Can you work these out from the model? Positions are in its coordinate system, mm. A direction names the side the tool comes from. Coordinates: 2 decimals unless noted, no trailing zeros. Order: outer loops, then holes, each group sorted by start corner. A loop starts at its lowest first (then second) coordinate and runs counter-clockwise, first axis right, second up. Notation, with made-up numbers: (19.25, 76) -> (67.25, 76) arc R27 cw to (67.25, 102) -> close; hole circle Ø9 at (73.25, 86). An arc over 180 degrees is marked (long way). Return JSON: item names as keys, results as strings. Group by question number.
1) For faces 1 (the cylindrical face through (-14.9, 7.5, 7.9)), 2 (the flat face through (-2, 8, 3.75)), 3 (the flat face through (-5, 3, 0)), which set-ups out of +Z, -Z, +X, -X, +Y, -Y let a thin tool reach every point of the face, with its end or its side?
2) If we section it at A-A, the plane z = 0: Please give me the cut outline in (x, y), then the cut area to 3 significant figures.
3) If I drill on probe 1 along Z at (x, y) = (0, 8.65) (3 decimals); probe 2 along X at (y, z) = (6.15, 0); probe 3 along Z at (x, y) = (-13.4, 6.9) (3 decimals), over which ranges is the centre line in solid material (lowest first)? Write a range as from..to.
4) If we section it at C-C, the plane y = 9: Please give me the cut outline in (x, z) (3 decimals), then the cut area to 3 significant figures.
5) If we section it at B-B, the plane x = -13.4: Please give me the cut outline in (y, z) (3 decimals), then the cut area to 3 significant figures.
6) For pin 1 (5 mm diameter, centred on x = -1, z = -0.5, fed in from -Y); pin 2 (1.5 mm diameter, centred on x = -13.5, z = -7.5, fed in from +Y); pin 3 (11.5 mm diameter, centred on x = -3, z = 1, fed in from -Y); pin 4 (2 mm diameter, centred on x = -6, z = -0.5, fed in from +Y), each with a flat end and sliding along its axis, tell me the tip position at first contact or that it passes through.
Autodesk Inventor part; units mm, degrees
ref_plane "YZ Plane" through (0, 0, 0) normal (1, 0, 0) x (0, 1, 0)
ref_plane "XZ Plane" through (0, 0, 0) normal (0, 1, 0) x (-1, 0, 0)
ref_plane "XY Plane" through (0, 0, 0) normal (0, 0, 1) x (1, 0, 0)
sketch "Sketch1" plane through (0, 0, 0) normal (0, 1, 0) x (-1, 0, 0)
  circle A0 centre (7.3, 0) radius 1.55
  circle A1 centre (0, 0) radius 1.55
  line L0 (0, 10.8163) -> (0, -10.8163)
  line L1 (6.335, 0) -> (-6.335, 0)
  line L2 (-3.05, 12.16) -> (16.95, 12.16)
  line L3 (16.95, 12.16) -> (16.95, -12.16)
  line L4 (16.95, -12.16) -> (-3.05, -12.16)
  line L5 (-3.05, -12.16) -> (-3.05, 12.16)
  dimension "d0" = 3.1
  dimension "d1" = 7.3
  dimension "d2" = 1.5
  dimension "d3" = 24.32
  dimension "d4" = 20
extrude "Extrusion1" add sketch "Sketch1" along normal blind 10
sketch "Sketch2" plane through (0, 0, 0) normal (0, -1, 0) x (1, 0, 0)
  line L0 (3.05, 5.16) -> (-11.68, 5.16)
  line L1 (-11.68, 5.16) -> (-11.68, -5.16)
  line L2 (-11.68, -5.16) -> (3.05, -5.16)
  line L3 (3.05, -5.16) -> (3.05, 5.16)
  circle A0 centre (0, 0) radius 1.55
  circle A1 centre (-7.3, 0) radius 1.55
  line L4 (0, 0) -> (-7.3, 0)
  line L5 (3.05, 12.16) -> (3.05, -12.16)
  dimension "d7" = 10.32
  dimension "d8" = 4.38
extrude "Extrusion2" cut sketch "Sketch2" against normal blind 3
sketch "Sketch3" plane through (0, 10, 0) normal (0, 1, 0) x (1, 0, 0)
  circle A0 centre (-7.3, 0) radius 1.55
  circle A1 centre (0, 0) radius 1.55
  arc A2 (3.05, -2.1817) -> (3.05, 2.1817) centre (0, 0) ccw
  arc A3 (-7.3, 3.75) -> (-7.3, -3.75) centre (-7.3, 0) ccw
  line L0 (3.05, -12.16) -> (3.05, 12.16)
  line L1 (-7.3, 3.75) -> (0, 3.75)
  line L2 (-7.3, -3.75) -> (0, -3.75)
  line L3 (3.05, -2.1817) -> (3.05, 2.1817)
  line L4 (3.05, -2.1817) -> (3.05, 2.1817)
  line L5 (0, -3.75) -> (3.05, -3.75)
  line L6 (0, 3.75) -> (3.05, 3.75)
  dimension "d11" = 7.5
extrude "Extrusion3" cut sketch "Sketch3" against normal blind 3 contours L0 L5 L2 A3 L1 L6
sketch "Sketch4" plane through (0, 10, 0) normal (0, 1, 0) x (1, 0, 0)
  line L0 (3.05, -12.16) -> (3.05, -3.75)
  line L1 (3.05, -3.75) -> (-7.3, -3.75)
  arc A0 (-7.3, 3.75) -> (-7.3, -3.75) centre (-7.3, 0) ccw
  line L2 (-7.3, 3.75) -> (3.05, 3.75)
  line L3 (3.05, 3.75) -> (3.05, -3.75)
  circle A1 centre (0, -7.955) radius 1.5
  circle A2 centre (-13.4, -7.955) radius 1.5
  line L4 (-16.95, 12.16) -> (-16.95, -12.16)
  line L5 (-16.95, 0) -> (3.05, 0)
  circle A3 centre (0, 7.955) radius 1.5
  circle A4 centre (-13.4, 7.955) radius 1.5
  line L6 (3.05, -7.955) -> (-16.95, -7.955)
  line L7 (3.05, 5.16) -> (3.05, 12.16)
  line L8 (3.05, 7.955) -> (-16.95, 7.955)
  line L9 (-11.05, 0) -> (-16.95, 0) construction
  point P0 (0, 0)
  dimension "d15" = 3
  dimension "d16" = 3
  dimension "d18" = 3.05
  dimension "d19" = 3.55
extrude "Extrusion4" cut sketch "Sketch4" against normal blind 5 contours L6 A1 | A1 L6 | L6 A2 | A2 L6 | L8 A3 | A3 L8 | L8 A4 | A4 L8
chamfer "Chamfer1" distance 0.5 angle 45 26 edges at (3.05, 10, 7.955) (-2.125, 10, 3.75) (-11.05, 10, 0) (-2.125, 10, -3.75) (3.05, 10, -7.955) (-6.95, 10, -12.16) (-16.95, 10, 0) (-6.95, 10, 12.16) (3.05, 5, 12.16) (3.05, 0, 8.66) (-6.95, 0, 12.16) (-16.95, 0, 0) (-6.95, 0, -12.16) (3.05, 0, -8.66) (3.05, 5, -12.16) (-16.95, 5, -12.16) (-16.95, 5, 12.16) (-11.68, 0, 0) (-4.315, 0, 5.16) (-4.315, 0, -5.16) (3.05, 1.5, 5.16) (3.05, 1.5, -5.16) (3.05, 3, 0) (3.05, 7, 0) (3.05, 8.5, 3.75) (3.05, 8.5, -3.75)
equation "\"d0\" = spacer_hole_diameter"
equation "\"d1\" = load_cell_hole_discance"
equation "\"load_cell_hole_discance\" = 7.3"
equation "\"spacer_hole_diameter\" = 3.1"
equation "\"load_cell_width\" = 9.32"
equation "\"load_cell_hole_edge\" = 4.18"
properties part number "load_cell_connector_bottom"
Result sheet:
{
 "1": {"face 1": "+Y", "face 2": "+X, +Y", "face 3": "+X, -Y"},
 "2": {"outline": "(-16.95, 0.5) -> (-16.45, 0) -> (-12.18, 0) -> (-11.68, 0.5) -> (-11.68, 3) -> (-8.85, 3) -> (-8.85, 7) -> (-11.05, 7) -> (-11.05, 9.5) -> (-11.55, 10) -> (-16.45, 10) -> (-16.95, 9.5) -> close; (-5.75, 3) -> (-1.55, 3) -> (-1.55, 7) -> (-5.75, 7) -> close; (1.55, 3) -> (2.55, 3) -> (3.05, 3.5) -> (3.05, 6.5) -> (2.55, 7) -> (1.55, 7) -> close", "area": "88.0 mm2"},
 "3": {"probe 1": "z = -12.16..-9.455, -6.455..-3.75, 3.75..6.455, 9.455..12.16", "probe 2": "x = -16.95..-8.85, -5.75..-1.55, 1.55..3.05", "probe 3": "z = -12.16..-9.455, -6.455..6.455, 9.455..12.16"},
 "4": {"outline": "(-16.95, -11.66) -> (-16.45, -12.16) -> (2.55, -12.16) -> (3.05, -11.66) -> (3.05, -4.25) -> (2.55, -3.75) -> (-7.3, -3.75) arc R3.75 cw to (-7.3, 3.75) -> (2.55, 3.75) -> (3.05, 4.25) -> (3.05, 11.66) -> (2.55, 12.16) -> (-16.45, 12.16) -> (-16.95, 11.66) -> close; hole circle Ø3 at (-13.4, -7.955); hole circle Ø3 at (-13.4, 7.955); hole circle Ø3 at (0, -7.955); hole circle Ø3 at (0, 7.955)", "area": "358 mm2"},
 "5": {"outline": "(0, -11.66) -> (0.5, -12.16) -> (9.5, -12.16) -> (10, -11.66) -> (10, -9.455) -> (5, -9.455) -> (5, -6.455) -> (10, -6.455) -> (10, 6.455) -> (5, 6.455) -> (5, 9.455) -> (10, 9.455) -> (10, 11.66) -> (9.5, 12.16) -> (0.5, 12.16) -> (0, 11.66) -> close", "area": "213 mm2"},
 "6": {"pin 1": "stops at y = 3", "pin 2": "stops at y = 5", "pin 3": "stops at y = 0", "pin 4": "stops at y = 7"}
}
